```python
from build123d import *

# Parameters (mm, degrees)
BOSS_EXTRUDE1_DEPTH = 92.28812
BOSS_EXTRUDE2_DEPTH = 66.46188
BOSS_EXTRUDE3_DEPTH = 307.975
BOSS_EXTRUDE4_DEPTH = 177.926
SKETCH6_W           = 25.148038513
SKETCH6_H           = 72.870812273
BOSS_EXTRUDE5_DEPTH = 307.975


with BuildPart() as part:
    # Sketch1 → Boss-Extrude1 (new body)
    with BuildSketch(Plane.ZY.offset(470.597286824)):
        Polygon((375.982707359, 100.269590084), (375.982707359, 15.687590084), (347.407707359, 15.687590084), (-308.166292641, 15.433590084), (-339.916292641, 15.433590084), (-339.916292641, 100.015590084), (-289.116292641, 100.015590084), (328.357707359, 100.269590084), align=None)
    extrude(amount=-BOSS_EXTRUDE1_DEPTH)

    # Sketch2 → Boss-Extrude2 (add)
    with BuildSketch(Plane(origin=(-378.309166646, 0, 0), x_dir=(0, 0, -1), z_dir=(1, 0, 0))):
        Polygon((-375.220707359, 18.862590084), (-344.232707359, 18.862590084), (-344.232707359, 15.687590084), (-325.182707359, 15.687590084), (-325.182707359, 97.094590084), (-375.220707359, 97.094590084), align=None)
        Polygon((-375.220707359, 100.269590084), (-375.220707359, 97.094590084), (-325.182707359, 97.094590084), (-325.182707359, 100.268284038), (-328.357707359, 100.269590084), align=None)
        with BuildLine():
            ThreePointArc((-375.982707359, 96.332590084), (-375.759522726, 96.871405452), (-375.220707359, 97.094590084))
            Line((-375.220707359, 97.094590084), (-375.220707359, 100.269590084))
            ThreePointArc((-375.220707359, 100.269590084), (-375.60352134, 100.250934436), (-375.982707359, 100.195144291))
            Line((-375.982707359, 100.195144291), (-375.982707359, 96.332590084))
        make_face()
        with BuildLine():
            ThreePointArc((-375.982707359, 19.624590084), (-375.759522726, 19.085774717), (-375.220707359, 18.862590084))
            Line((-375.220707359, 18.862590084), (-375.220707359, 97.094590084))
            ThreePointArc((-375.220707359, 97.094590084), (-375.759522726, 96.871405452), (-375.982707359, 96.332590084))
            Line((-375.982707359, 96.332590084), (-375.982707359, 19.624590084))
        make_face()
        Polygon((-344.232707359, 15.687590084), (-344.232707359, 18.862590084), (-375.220707359, 18.862590084), (-375.220707359, 15.687590084), (-347.407707359, 15.687590084), align=None)
        with BuildLine():
            Line((-375.220707359, 15.687590084), (-375.220707359, 18.862590084))
            ThreePointArc((-375.220707359, 18.862590084), (-375.759522726, 19.085774717), (-375.982707359, 19.624590084))
            Line((-375.982707359, 19.624590084), (-375.982707359, 15.762035878))
            ThreePointArc((-375.982707359, 15.762035878), (-375.60352134, 15.706245733), (-375.220707359, 15.687590084))
        make_face()
    extrude(amount=BOSS_EXTRUDE2_DEPTH)

    # Sketch3 → Boss-Extrude3 (add)
    with BuildSketch(Plane(origin=(-378.309166646, 0, 0), x_dir=(0, 0, -1), z_dir=(1, 0, 0))):
        Polygon((289.116292641, 100.015590084), (289.116292641, 25.212590084), (57.341292641, 25.212590084), (57.341292641, 22.037590084), (289.116292641, 22.037590084), (289.116292641, 15.440970945), (308.166292641, 15.433590084), (339.916292641, 15.433590084), (339.916292641, 100.015590084), align=None)
    extrude(amount=BOSS_EXTRUDE3_DEPTH)

    # Sketch4 → Boss-Extrude4 (add)
    with BuildSketch(Plane(origin=(-378.309166646, 0, 0), x_dir=(0, 0, -1), z_dir=(1, 0, 0))):
        with BuildLine():
            ThreePointArc((44.31439752, 41.659090084), (35.270733675, 63.492426094), (13.437397726, 72.536090084))
            ThreePointArc((13.437397726, 72.536090084), (-5.359329042, 66.155461235), (-16.387494219, 49.65064574))
            ThreePointArc((-16.387494219, 49.65064574), (-15.318667207, 30.412852027), (-3.052669821, 15.554170853))
            Line((-3.052669821, 15.554170853), (29.907231382, 15.541400647))
            ThreePointArc((29.907231382, 15.541400647), (38.295788177, 23.343808407), (43.262289258, 33.667534429))
            ThreePointArc((43.262289258, 33.667534429), (44.050240504, 37.628832847), (44.31439752, 41.659090084))
        make_face()
        with BuildLine():
            ThreePointArc((-22.8539205, 49.65064574), (-33.882085595, 66.155461173), (-52.678812238, 72.536090084))
            ThreePointArc((-52.678812238, 72.536090084), (-74.512148435, 63.492426054), (-83.555812238, 41.659089763))
            ThreePointArc((-83.555812238, 41.659089763), (-83.291655202, 37.628832688), (-82.503703977, 33.667534429))
            ThreePointArc((-82.503703977, 33.667534429), (-77.55849945, 23.372748372), (-69.209387458, 15.579803056))
            Line((-69.209387458, 15.579803056), (-36.168450647, 15.567001453))
            ThreePointArc((-36.168450647, 15.567001453), (-23.918377136, 30.424033264), (-22.8539205, 49.65064574))
        make_face()
        with BuildLine():
            Line((13.437397726, 72.536090084), (-52.678812238, 72.536090084))
            ThreePointArc((-52.678812238, 72.536090084), (-33.882085595, 66.155461173), (-22.8539205, 49.65064574))
            ThreePointArc((-22.8539205, 49.65064574), (-23.918377136, 30.424033264), (-36.168450647, 15.567001453))
            Line((-36.168450647, 15.567001453), (-3.052669821, 15.554170853))
            ThreePointArc((-3.052669821, 15.554170853), (-15.318667207, 30.412852027), (-16.387494219, 49.65064574))
            ThreePointArc((-16.387494219, 49.65064574), (-5.359329042, 66.155461235), (13.437397726, 72.536090084))
        make_face()
        with BuildLine():
            ThreePointArc((-52.678812238, 10.782090084), (-44.083938524, 12.002433583), (-36.168450647, 15.567001453))
            Line((-36.168450647, 15.567001453), (-69.209387458, 15.579803056))
            ThreePointArc((-69.209387458, 15.579803056), (-61.285175681, 12.005765865), (-52.678812238, 10.782090084))
        make_face()
        with BuildLine():
            Line((-3.052669821, 15.554170853), (-36.168450647, 15.567001453))
            ThreePointArc((-36.168450647, 15.567001453), (-44.083938524, 12.002433583), (-52.678812238, 10.782090084))
            Line((-52.678812238, 10.782090084), (13.437397518, 10.782090084))
            ThreePointArc((13.437397518, 10.782090084), (4.854054992, 11.999094129), (-3.052669821, 15.554170853))
        make_face()
        with BuildLine():
            Line((29.907231382, 15.541400647), (-3.052669821, 15.554170853))
            ThreePointArc((-3.052669821, 15.554170853), (4.854054992, 11.999094129), (13.437397518, 10.782090084))
            ThreePointArc((13.437397518, 10.782090084), (22.009247734, 11.995770768), (29.907231382, 15.541400647))
        make_face()
        with BuildLine():
            Line((44.31439752, 10.782090084), (44.31439752, 15.535818637))
            Line((44.31439752, 15.535818637), (29.907231382, 15.541400647))
            ThreePointArc((29.907231382, 15.541400647), (22.009247734, 11.995770768), (13.437397518, 10.782090084))
            Line((13.437397518, 10.782090084), (44.31439752, 10.782090084))
        make_face()
        with BuildLine():
            Line((-69.209387458, 15.579803056), (-83.555812238, 15.585361532))
            Line((-83.555812238, 15.585361532), (-83.555812238, 10.782090084))
            Line((-83.555812238, 10.782090084), (-52.678812238, 10.782090084))
            ThreePointArc((-52.678812238, 10.782090084), (-61.285175681, 12.005765865), (-69.209387458, 15.579803056))
        make_face()
        with BuildLine():
            ThreePointArc((-82.503703977, 33.667534429), (-83.291655202, 37.628832688), (-83.555812238, 41.659089763))
            Line((-83.555812238, 41.659089763), (-83.555812238, 15.585361532))
            Line((-83.555812238, 15.585361532), (-69.209387458, 15.579803056))
            ThreePointArc((-69.209387458, 15.579803056), (-77.55849945, 23.372748372), (-82.503703977, 33.667534429))
        make_face()
        with BuildLine():
            Line((-52.678812238, 72.536090084), (-83.555812238, 72.536090084))
            Line((-83.555812238, 72.536090084), (-83.555812238, 41.659089763))
            ThreePointArc((-83.555812238, 41.659089763), (-74.512148435, 63.492426054), (-52.678812238, 72.536090084))
        make_face()
        with BuildLine():
            Line((44.31439752, 72.536090084), (13.437397726, 72.536090084))
            ThreePointArc((13.437397726, 72.536090084), (35.270733675, 63.492426094), (44.31439752, 41.659090084))
            Line((44.31439752, 41.659090084), (44.31439752, 72.536090084))
        make_face()
        with BuildLine():
            Line((44.31439752, 15.535818637), (44.31439752, 41.659090084))
            ThreePointArc((44.31439752, 41.659090084), (44.050240504, 37.628832847), (43.262289258, 33.667534429))
            ThreePointArc((43.262289258, 33.667534429), (38.295788177, 23.343808407), (29.907231382, 15.541400647))
            Line((29.907231382, 15.541400647), (44.31439752, 15.535818637))
        make_face()
    extrude(amount=BOSS_EXTRUDE4_DEPTH)

    # Sketch6 → Boss-Extrude5 (add)
    with BuildSketch(Plane(origin=(-378.309166646, 0, 0), x_dir=(0, 0, -1), z_dir=(1, 0, 0))):
        with Locations((-123.855467844, 59.050323619)):
            Rectangle(SKETCH6_W, SKETCH6_H)
    extrude(amount=BOSS_EXTRUDE5_DEPTH)

    # Mirror1: part across plane


with BuildPart() as part_1:
    add(part.part)
    add(part.part.mirror(Plane(origin=(-70.334166646, 0, 0), x_dir=(0, 0, 1), z_dir=(1, 0, 0))))


solid = part_1.part
```
CAD build for the part. Positions are in the model's coordinates, mm. A direction names the side the tool comes from. Round coordinates to 2 decimals unless told otherwise and drop trailing zeros. Order: outer loops, then holes, each group sorted by start corner. A loop starts at its lowest first (then second) coordinate and runs counter-clockwise, first axis right, second up.
Item 1: Mould opens along Z. For faces 4 (the face through (-392, 59, 375.983)), 5 (the face through (-291, 10.782, 21)), 6 (the face through (59.715, 42, 21)) say: pulls with the +Z half, pulls with the -Z half, needs draft (parallel to the pull), parting line crosses it, or undercut.
Item 2: Saw through at A-A on x = -349. Write the cut outline in (y, z).
Item 3: Saw through at C-C on x = -135. Write the cut outline in (y, z), then the cut area to 3 significant figures.
Item 4: Saw through at B-B on y = 83.5. Write the cut outline in (x, z), then the cut area to 3 significant figures.
Item 5: Probe line 1 along Z through (x, y) = (-339, 19); line 2 along Z through (x, y) = (150, 29); line 3 along Z through (x, y) = (223.5, 57.5). List the from-to ranges inside material, lowest first.
Item 6: Saw through at D-D on z = -8. Write the cut outline in (x, y), then the cut area to 3 significant figures.
Item 7: Pin check, flat tips, straight feed: pin 1 (1 mm diameter, centred on x = -177, y = 23.5, fed in from +Z); pin 2 (2 mm diameter, centred on x = -90, y = 19, fed in from +Z). Stop position of each tip, or through.
Item 8: Tool access for faces 1 (the face through (-66, 59, 136.429)), 2 (the face through (150, 72.536, 19)), 3 (the face through (-66, 22.615, 124)): list every direction of +Z, -Z, +X, -X, +Y, -Y with a clear straight run to the whole face (end or side of a thin tool).
Reported:
1. face 4: pulls with the +Z half
1. face 5: needs draft
1. face 6: undercut
2. outline: (10.78, -44.31) - (72.54, -44.31) - (72.54, 83.56) - (10.78, 83.56) - close; (15.43, -339.92) - (100.02, -339.92) - (100.02, -289.12) - (25.21, -289.12) - (25.21, -57.34) - (22.04, -57.34) - (22.04, -289.12) - (15.44, -289.12) - (15.43, -308.17) - close; (15.69, 325.18) - (100.27, 325.18) - (100.27, 328.36) - (100.27, 375.22) arc R3.94 ccw to (100.2, 375.98) - (15.76, 375.98) arc R3.94 ccw to (15.69, 375.22) - close; (22.61, 111.28) - (95.49, 111.28) - (95.49, 136.43) - (22.61, 136.43) - close
3. outline: (15.43, -339.92) - (100.02, -339.92) - (100.02, -289.12) - (25.21, -289.12) - (25.21, -57.34) - (22.04, -57.34) - (22.04, -289.12) - (15.44, -289.12) - (15.43, -308.17) - close; (22.61, 111.28) - (95.49, 111.28) - (95.49, 136.43) - (22.61, 136.43) - close
3. area: 6,870 mm2
4. outline: (-470.6, -339.92) - (329.93, -339.92) - (329.93, 375.98) - (171.18, 375.98) - (171.18, 325.18) - (237.64, 325.18) - (237.64, 136.43) - (-378.31, 136.43) - (-378.31, 325.18) - (-311.85, 325.18) - (-311.85, 375.98) - (-470.6, 375.98) - close; hole (-378.31, -289.12) - (237.64, -289.12) - (237.64, 111.28) - (-378.31, 111.28) - close
4. area: 186,000 mm2
5. line 1: z = -339.92 to -289.12, -44.31 to 83.56, 325.18 to 375.98
5. line 2: z = -339.92 to -289.12, -44.31 to 83.56, 111.28 to 136.43
5. line 3: z = -339.92 to -289.12, -44.31 to 83.56, 111.28 to 136.43, 325.18 to 375.98
6. outline: (-470.6, 15.55) - (-378.31, 15.55) - (-378.31, 10.78) - (-200.38, 10.78) - (-200.38, 72.54) - (-378.31, 72.54) - (-378.31, 100.13) - (-470.6, 100.13) - close; (59.71, 10.78) - (237.64, 10.78) - (237.64, 15.55) - (329.93, 15.55) - (329.93, 100.13) - (237.64, 100.13) - (237.64, 72.54) - (59.71, 72.54) - close
6. area: 37,600 mm2
7. pin 1: stops at z = 136.43
7. pin 2: stops at z = -289.12
8. face 1: +Y, -Y
8. face 2: +Y
8. face 3: -Y
